```python
from build123d import *

# Parameters (mm, degrees)
F0_W     = 120
F0_H     = 30
F0_R     = 1.35
F1_DEPTH = 5
F2_SIZE  = 2.5
F3_R     = 1


with BuildPart() as f1:
    # F0 (on Top) → F1 (new body)
    with BuildSketch(Plane.XY):
        with Locations((0, 7)):
            Rectangle(F0_W, F0_H)
        with Locations((-50, 0)):
            Circle(F0_R, mode=Mode.SUBTRACT)
        with Locations((-30, 0)):
            Circle(F0_R, mode=Mode.SUBTRACT)
        with Locations((-10, 0)):
            Circle(F0_R, mode=Mode.SUBTRACT)
        with Locations((10, 0)):
            Circle(F0_R, mode=Mode.SUBTRACT)
        with Locations((30, 0)):
            Circle(F0_R, mode=Mode.SUBTRACT)
        with Locations((50, 0)):
            Circle(F0_R, mode=Mode.SUBTRACT)
    extrude(amount=F1_DEPTH)

    # F2
    f2_edges = [f1.edges().sort_by_distance(p)[0] for p in [
        (-51.35, 0, 0),
        (-31.35, 0, 0),
        (-11.35, 0, 0),
        (8.65, 0, 0),
        (28.65, 0, 0),
        (48.65, 0, 0),
    ]]
    chamfer(f2_edges, length=F2_SIZE)

    # F3
    f3_edges = [f1.edges().sort_by_distance(p)[0] for p in [
        (-60, 7, 5),
        (0, -8, 5),
        (60, 7, 5),
        (0, 22, 5),
        (60, 22, 2.5),
        (60, -8, 2.5),
        (-60, -8, 2.5),
        (-60, 22, 2.5),
    ]]
    fillet(f3_edges, radius=F3_R)


solid = f1.part
```
Check sheet for the modelled part. Datum: model origin and axes. Units: mm. Give positions to 0.01 mm unless a question says otherwise; leave off trailing zeros. Loops run counter-clockwise (first coordinate to the right, second up) from the corner with the lowest first, then second, coordinate; pieces in that order, holes last. Notation, with made-up numbers: (51, 22) - (91, 22) arc R10 cw to (91, 33) - close; hole circle Ø4 at (66.25, 61). An arc over 180 degrees is marked (long way). One line per question, with ' | ' between items. Start each with the question number.
1. Material ranges on line 1 along Y through (x, z) = (-30, 3.2); line 2 along Y through (x, z) = (-50.5, 4.75); line 3 along Y through (x, z) = (13, 4.6), recorded low to high. Write a range as [from, to].
2. Gauge pin test, flat ends, axial feed: pin 1 Ø2 at (x, y) = (-30, 0) entering from +Z; pin 2 Ø4.5 at (x, y) = (-50, 0) entering from -Z; pin 3 Ø3 at (x, y) = (-10, 0) entering from -Z. Record the tip position at first contact, or that the pin passes through.
3. Cross-section at B-B, the plane z = 1.65. Enter the section's corners in (x, y).
4. Cross-section at A-A, the plane x = 10. Enter the section's corners in (y, z).
5. Draft check along X on faces 1 (the flat face through (-60, 7, 2)), 2 (the conical face through (-11.505, 0.066, 2.344)), 3 (the flat face through (-1, -8, 2)), 4 (the cylindrical face through (48.65, 0.06, 3.73)). Enter one of: released by +X, released by -X, zero draft, split by the parting line, or undercut.
6. Cross-section at C-C, the plane y = 0. Give the number of separate pieces and of enclosed holes in the cut face, plus the area to 3 significant figures.
Check result:
1) line 1: y = [-8, -1.35], [1.35, 22] | line 2: y = [-7.66, -1.25], [1.25, 21.66] | line 3: y = [-7.8, 21.8]
2) pin 1: passes through | pin 2: stops at z = 1.6 | pin 3: stops at z = 2.35
3) outline: (-60, -7) arc R1 ccw to (-59, -8) - (59, -8) arc R1 ccw to (60, -7) - (60, 21) arc R1 ccw to (59, 22) - (-59, 22) arc R1 ccw to (-60, 21) - close; hole circle Ø4.4 at (-50, 0); hole circle Ø4.4 at (-30, 0); hole circle Ø4.4 at (-10, 0); hole circle Ø4.4 at (10, 0); hole circle Ø4.4 at (30, 0); hole circle Ø4.4 at (50, 0)
4) outline: (-8, 0) - (-3.85, 0) - (-1.35, 2.5) - (-1.35, 5) - (-7, 5) arc R1 ccw to (-8, 4) - close; (1.35, 2.5) - (3.85, 0) - (22, 0) - (22, 4) arc R1 ccw to (21, 5) - (1.35, 5) - close
5) face 1: released by -X | face 2: undercut | face 3: zero draft | face 4: undercut
6) separate pieces: 7 | enclosed holes: 0 | area: 481 mm2
